Check sheet for the modelled part. Datum: model origin and axes. Units: mm. Coordinates: 2 decimals unless noted, no trailing zeros. Write each loop counter-clockwise with the first axis right and the second up, starting at its lowest first coordinate (ties: lowest second). Pieces come first, ordered by that corner, then holes. Notation, with made-up numbers: M -38,-11 L 15,-11 A29 ccw 15,18 Z; hole C 69.25,76.5 d5. An arc over 180 degrees is marked long. Answer as CSV lines item,"result". Start each with the question number.
1) Section check D-D (x = 12). Record the cut outline in (y, z) (3 decimals), and give its area (3 significant figures).
2) Section check C-C (x = 0). Record the cut outline in (y, z) (3 decimals).
3) Section check A-A (z = 0). Record the cut outline in (x, y) (3 decimals).
4) Material ranges on L1, parallel to X at y = 1.65, z = 0 (3 decimals); L2, parallel to Z at x = 0, y = 1.6; L3, parallel to X at y = 2.25, z = 7.5 (3 decimals), recorded low to high. Write a range as [from, to].
5) Section check B-B (y = 1.8). Record the cut outline in (x, z) (3 decimals).
6) Go/stop test with flat-tipped pins: pin 1 Ø0.7 at (y, z) = (2, 42) entering from -X; pin 2 Ø1 at (x, y) = (18, 1.5) entering from +Z (3 decimals); pin 3 Ø1.5 at (x, y) = (10.5, 2) entering from +Z. Record where each tip stops, or that it passes through.
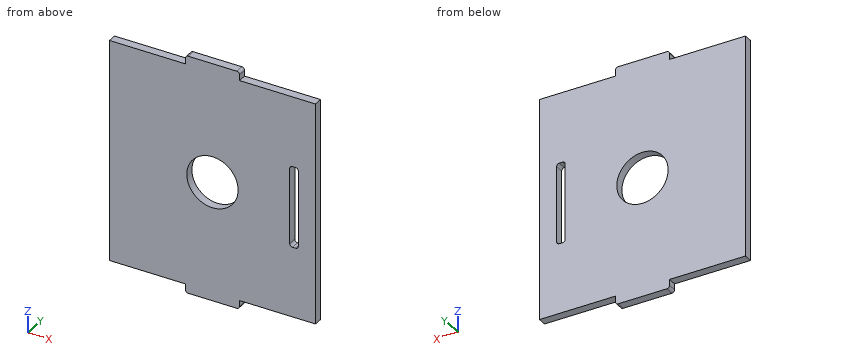
from build123d import *

# Parameters (mm, degrees)
BOSS_EXTRUDE1_DEPTH = 3.175
SKETCH2_R           = 9.5
SKETCH2_W           = 3.175
SKETCH2_H           = 30
CUT_EXTRUDE1_DEPTH  = 4.175
FILLET1_R           = 1


with BuildPart() as part:
    # Sketch1 → Boss-Extrude1 (new body)
    with BuildSketch(Plane(origin=(0, 0, 0), x_dir=(1, 0, 0), z_dir=(0, 1, 0))):
        Polygon((-38.1, -40.925), (-10, -40.925), (-10, -44.1), (10, -44.1), (10, -40.925), (38.1, -40.925), (38.1, 40.925), (10, 40.925), (10, 44.1), (-10, 44.1), (-10, 40.925), (-38.1, 40.925), align=None)
    extrude(amount=BOSS_EXTRUDE1_DEPTH)

    # Sketch2 → Cut-Extrude1 (cut, through all)
    with BuildSketch(Plane(origin=(0, 3.175, 0), x_dir=(1, 0, 0), z_dir=(0, 1, 0))):
        Circle(SKETCH2_R)
        with Locations((30.1625, 0)):
            Rectangle(SKETCH2_W, SKETCH2_H)
    extrude(amount=-CUT_EXTRUDE1_DEPTH, mode=Mode.SUBTRACT)

    # Fillet1
    fillet1_edges = [part.edges().sort_by_distance(p)[0] for p in [
        (10, 1.5875, 44.1),
        (-10, 1.5875, 44.1),
        (-10, 1.5875, -44.1),
        (10, 1.5875, -44.1),
        (28.575, 1.5875, 15),
        (28.575, 1.5875, -15),
        (31.75, 1.5875, -15),
        (31.75, 1.5875, 15),
    ]]
    fillet(fillet1_edges, radius=FILLET1_R)


solid = part.part
Results found:
1,outline,"M 0,-40.925 L 3.175,-40.925 L 3.175,40.925 L 0,40.925 Z"
1,area,"260 mm2"
2,outline,"M 0,-44.1 L 3.175,-44.1 L 3.175,-9.5 L 0,-9.5 Z; M 0,9.5 L 3.175,9.5 L 3.175,44.1 L 0,44.1 Z"
3,outline,"M -38.1,0 L -9.5,0 L -9.5,3.175 L -38.1,3.175 Z; M 9.5,0 L 28.575,0 L 28.575,3.175 L 9.5,3.175 Z; M 31.75,0 L 38.1,0 L 38.1,3.175 L 31.75,3.175 Z"
4,L1,"x = [-38.1, -9.5], [9.5, 28.575], [31.75, 38.1]"
4,L2,"z = [-44.1, -9.5], [9.5, 44.1]"
4,L3,"x = [-38.1, -5.831], [5.831, 28.575], [31.75, 38.1]"
5,outline,"M -38.1,-40.925 L -10,-40.925 L -10,-43.1 A1 ccw -9,-44.1 L 9,-44.1 A1 ccw 10,-43.1 L 10,-40.925 L 38.1,-40.925 L 38.1,40.925 L 10,40.925 L 10,43.1 A1 ccw 9,44.1 L -9,44.1 A1 ccw -10,43.1 L -10,40.925 L -38.1,40.925 Z; hole C 0,0 d19; hole M 28.575,-14 A1 ccw 29.575,-15 L 30.75,-15 A1 ccw 31.75,-14 L 31.75,14 A1 ccw 30.75,15 L 29.575,15 A1 ccw 28.575,14 Z"
6,pin 1,"stops at x = -10"
6,pin 2,"stops at z = 40.925"
6,pin 3,"stops at z = 43.76"
